Could you check a few things on this model? Use its own coordinates, in mm. Face numbers are marked on the shaded views. Round coordinates to 2 decimals unless told otherwise and drop trailing zeros. Write each loop counter-clockwise with the first axis right and the second up, starting at its lowest first coordinate (ties: lowest second). Pieces come first, ordered by that corner, then holes. Notation, with made-up numbers: (12, 60.5) - (43, 60.5) arc R15 cw to (43, 71.5) - close; hole circle Ø3 at (11, 77.25). An arc over 180 degrees is marked (long way). Write each question's results on one line, items separated by ' | '. Start each with the question number.
(1) Imagine slicing it at C-C on z = 1.75. Write out the boundary of the cut face in (x, y), then the cut area to 3 significant figures.
(2) For P1, Ø1.5, axis at y = -3, z = 2, coming from the +X side; P2, Ø1.5, axis at y = 4, z = 4, coming from the -X side; P3, Ø1.5, axis at x = 2.5, z = 5.5, coming from the +Y side, each with a flat end and sliding along its axis, tell me the tip position at first contact or that it passes through.
(3) Imagine slicing it at A-A on x = 0. Write out the boundary of the cut face in (y, z).
(4) Imagine slicing it at D-D on z = 0.5. Write out the boundary of the cut face in (x, y).
(5) Please list where these lines run through material, in increasing order: line 1 (Y direction, x = 0, z = 7.25); line 2 (X direction, y = -0.25, z = 1); line 3 (Y direction, x = 4.5, z = 7). Write a range as [from, to].
(6) Thinking about a two-plate mould opening in X: for the marked faces 1, 2 and 3, which applies, +X half, -X half, draft (parallel to the pull), parting line (faces both ways), or undercut?
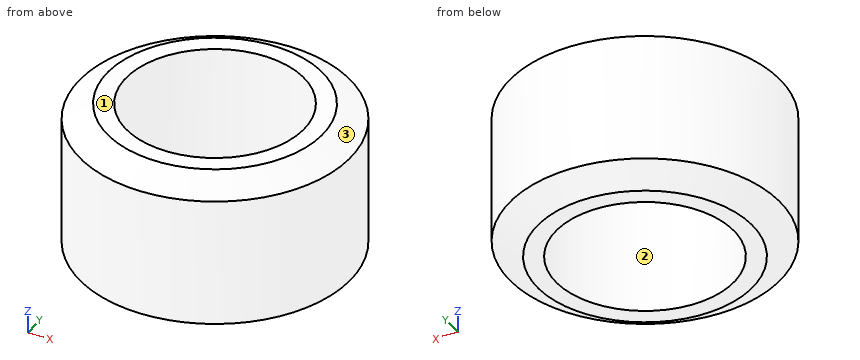
```python
from build123d import *

# Parameters (mm, degrees)
ESQUISSE1_R        = 7.6
ESQUISSE1_R_2      = 5
BOSS_EXTRU_1_DEPTH = 9
CHANFREIN5_SIZE    = 0.9
CHANFREIN5_SIZE2   = 1.558845727
CHANFREIN9_SIZE    = 0.9
CHANFREIN9_SIZE2   = 1.558845727


with BuildPart() as part:
    # Esquisse1 → Boss.-Extru.1 (new body)
    with BuildSketch(Plane.XY):
        Circle(ESQUISSE1_R)
        Circle(ESQUISSE1_R_2, mode=Mode.SUBTRACT)
    extrude(amount=BOSS_EXTRU_1_DEPTH)

    # Chanfrein5
    chanfrein5_edges = [part.edges().sort_by_distance(p)[0] for p in [
        (-7.6, 0, 9),
    ]]
    chanfrein5_side = [part.faces().sort_by_distance(p)[0] for p in [
        (-7.6, 0, 4.5),
    ]]
    chamfer(chanfrein5_edges, length=CHANFREIN5_SIZE, length2=CHANFREIN5_SIZE2, reference=chanfrein5_side[0])

    # Chanfrein9
    chanfrein9_edges = [part.edges().sort_by_distance(p)[0] for p in [
        (-7.6, 0, 0),
    ]]
    chanfrein9_side = [part.faces().sort_by_distance(p)[0] for p in [
        (-7.6, 0, 4.05),
    ]]
    chamfer(chanfrein9_edges, length=CHANFREIN9_SIZE, length2=CHANFREIN9_SIZE2, reference=chanfrein9_side[0])


solid = part.part
```
Response:
1) outline: circle Ø15.2 at (0, 0); hole circle Ø10 at (0, 0) | area: 103 mm²
2) P1: x = 7.26 | P2: x = -6.87 | P3: y = 7.4
3) outline: (-7.6, 0.9) - (-6.04, 0) - (-5, 0) - (-5, 9) - (-6.04, 9) - (-7.6, 8.1) - close; (5, 0) - (6.04, 0) - (7.6, 0.9) - (7.6, 8.1) - (6.04, 9) - (5, 9) - close
4) outline: circle Ø13.81 at (0, 0); hole circle Ø10 at (0, 0)
5) line 1: [-7.6, -5], [5, 7.6] | line 2: [-7.6, -4.99], [4.99, 7.6] | line 3: [-6.12, -2.18], [2.18, 6.12]
6) face 1: draft | face 2: undercut | face 3: parting line
